```python
from build123d import *

# Parameters (mm, degrees)
SKETCH1_W           = 120
SKETCH1_H           = 120
BOSS_EXTRUDE1_DEPTH = 5
SKETCH1_3_W         = 120
SKETCH1_3_H         = 120
SKETCH1_3_W_2       = 116
SKETCH1_3_H_2       = 116
BOSS_EXTRUDE2_DEPTH = 130
BOSS_EXTRUDE3_DEPTH = 57.5
SKETCH4_W           = 120
SKETCH4_H           = 5
BOSS_EXTRUDE4_DEPTH = 118
SKETCH5_R           = 26
CUT_EXTRUDE1_DEPTH  = 10


with BuildPart() as part:
    # Sketch1 → Boss-Extrude1 (new body)
    with BuildSketch(Plane(origin=(0, 0, 0), x_dir=(1, 0, 0), z_dir=(0, 1, 0))):
        Rectangle(SKETCH1_W, SKETCH1_H)
    extrude(amount=BOSS_EXTRUDE1_DEPTH)

    # Sketch1<3> → Boss-Extrude2 (add)
    with BuildSketch(Plane(origin=(0, 0, 0), x_dir=(1, 0, 0), z_dir=(0, 1, 0))):
        Rectangle(SKETCH1_3_W, SKETCH1_3_H)
        Rectangle(SKETCH1_3_W_2, SKETCH1_3_H_2, mode=Mode.SUBTRACT)
    extrude(amount=BOSS_EXTRUDE2_DEPTH)

    # Sketch2 → Boss-Extrude3 (add, symmetric)
    with BuildSketch(Plane.XY):
        Polygon((60, 130), (102.868257487, 105.25), (101.368257487, 102.651923789), (60, 126.535898385), align=None)
    boss_extrude3 = extrude(amount=BOSS_EXTRUDE3_DEPTH, both=True)

    # Mirror1: Boss-Extrude3 across plane
    add(boss_extrude3.mirror(Plane(origin=(0, 0, 0), x_dir=(0, 0, 1), z_dir=(1, 0, 0))))

    # Sketch4 → Boss-Extrude4 (add)
    with BuildSketch(Plane.XY.offset(-58)):
        with Locations((0, 67.5)):
            Rectangle(SKETCH4_W, SKETCH4_H)
    extrude(amount=BOSS_EXTRUDE4_DEPTH)

    # Sketch5 → Cut-Extrude1 (cut)
    with BuildSketch(Plane(origin=(0, 70, 0), x_dir=(1, 0, 0), z_dir=(0, 1, 0))):
        with Locations((28, 28)):
            Circle(SKETCH5_R)
        with Locations((-26, 28)):
            Circle(SKETCH5_R)
        with Locations((28, -28)):
            Circle(SKETCH5_R)
        with Locations((-26, -28)):
            Circle(SKETCH5_R)
    extrude(amount=-CUT_EXTRUDE1_DEPTH, mode=Mode.SUBTRACT)


solid = part.part
```
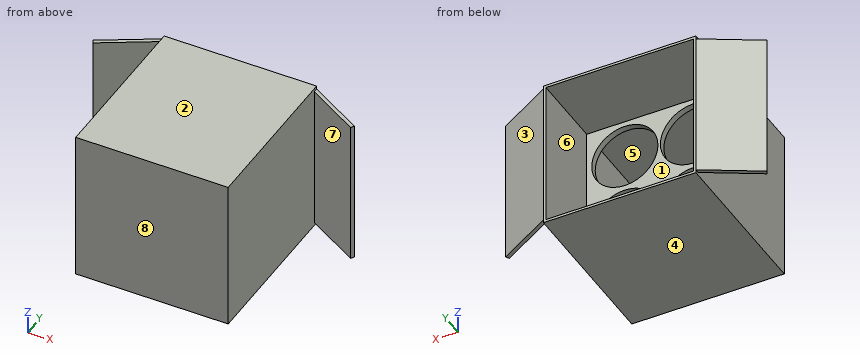
Source: CAD feature listing. Evaluate the final solid. Frame: model axes, mm. Face numbers are marked on the shaded views. A direction names the side the tool comes from. Coordinates: 2 decimals unless noted, no trailing zeros. Order: outer loops, then holes, each group sorted by start corner. A loop starts at its lowest first (then second) coordinate and runs counter-clockwise, first axis right, second up. Notation, with made-up numbers: M -1.75,0.25 L 11.25,0.25 A21 ccw 11.25,38.25 Z; hole C 58.5,6.5 d7. An arc over 180 degrees is marked long. Write each question's results on one line, items separated by ' | '. Start each with the question number.
1) Line query: line 1 (X direction, y = 68.35, z = 28); line 2 (Z direction, x = -26, y = 66.2); line 3 (X direction, y = 15, z = -55). Output: solid intervals per line, ascending. Write a range as from..to.
2) Contact query for flat-ended pins moving along their axis: pin 1 Ø13.5 at (x, y) = (76.5, 115.5) entering from +Z; pin 2 Ø5 at (y, z) = (25, -12.5) entering from -X; pin 3 Ø22 at (x, y) = (-88, 110) entering from -Z. Output: stop coordinate, or through.
3) Section query D-D (x = -23.5). Return the cut outline in (y, z).
4) Draft query along X for the marked faces 1, 2 and 3. Return one class per face: released by +X, released by -X, zero draft, split by the parting line, or undercut.
5) Access query for the marked faces 4, 5, 6, 7 and 8. Directions: +Z, -Z, +X, -X, +Y, -Y. A direction counts if a zero-diameter tool reaches every point of the face in a straight line with its end or side. Return the directions, or none.
6) Section query A-A (z = 28). Return the cut outline in (x, y), plus the area to 3 significant figures.
7) Section query C-C (x = 28). Return the cut outline in (y, z).
8) Section query B-B (y = 78.5). Return the cut outline in (x, z), plus the area to 3 significant figures.
Answers:
1) line 1: x = -60..-52, 0..2, 54..60 | line 2: z = -60..-54, -2..2, 54..60 | line 3: x = -60..-58, 58..60
2) pin 1: stops at z = 57.5 | pin 2: stops at x = -60 | pin 3: stops at z = -57.5
3) outline: M 0,-60 L 130,-60 L 130,-58 L 70,-58 L 70,-53.88 L 65,-53.88 L 65,-58 L 5,-58 L 5,58 L 65,58 L 65,53.88 L 70,53.88 L 70,58 L 130,58 L 130,60 L 0,60 Z; M 65,-2.12 L 70,-2.12 L 70,2.12 L 65,2.12 Z
4) face 1: undercut | face 2: zero draft | face 3: released by +X
5) face 4: -Z, +X, -X, +Y, -Y | face 5: none | face 6: +Y | face 7: +Z, -Z, -Y | face 8: +Z, -Z, +X, -X, -Y
6) outline: M -102.87,105.25 L -101.37,102.65 L -60,126.54 L -60,0 L 60,0 L 60,126.54 L 101.37,102.65 L 102.87,105.25 L 60,130 L 58,130 L 58,70 L 54,70 L 54,65 L 58,65 L 58,5 L -58,5 L -58,65 L -52,65 L -52,70 L -58,70 L -58,130 L -60,130 Z; M 0,65 L 2,65 L 2,70 L 0,70 Z | area: 1,450 mm^2
7) outline: M 0,-60 L 130,-60 L 130,-58 L 70,-58 L 70,-54 L 65,-54 L 65,-58 L 5,-58 L 5,58 L 65,58 L 65,54 L 70,54 L 70,58 L 130,58 L 130,60 L 0,60 Z; M 65,-2 L 70,-2 L 70,2 L 65,2 Z
8) outline: M -60,-60 L 60,-60 L 60,60 L -60,60 Z; hole M -58,-58 L 58,-58 L 58,58 L -58,58 Z | area: 944 mm^2
